from build123d import *

# Parameters (mm, degrees)
F6_R      = 38.8798944489
F7_DEPTH  = 25.146
F9_DEPTH  = 26.67
F10_W     = 18.4118933976
F10_H     = 2.2933566943
F11_DEPTH = 23.368


# Not quite as in the source:
# - a fillet or chamfer that OpenCascade refuses, or shapes differently, is made with other operations: its cross-section is extruded or revolved along the edge and cut away or added


with BuildPart() as f2:
    # F0 (on Front) → F2 (revolve)
    with BuildSketch(Plane.XZ):
        with BuildLine():
            ThreePointArc((-70.200012, 0), (-35.7013462561, 9.759799439), (0, 13.050012))
            Line((0, 13.050012), (0, 19.05))
            ThreePointArc((0, 19.05), (-39.272581084, 14.215324336), (-76.2, 0))
            Line((-76.2, 0), (-70.200012, 0))
        make_face()
    revolve(axis=Axis((0, 0, 24.1573229432), (0, 0, 1)))

    # F3: fillet of radius 2 on 1 edges, made by hand

    # F3_s1 → F3_t2 (revolve, cut)
    with BuildSketch(Plane.XZ):
        with BuildLine():
            ThreePointArc((-69.7074569816, 3.2775780346), (-70.8242638288, 1.7696123233), (-70.200012, 0))
            Line((-70.200012, 0), (-76.2, 0))
            ThreePointArc((-76.2, 0), (-72.9721325586, 1.6752455717), (-69.7074569816, 3.2775780346))
        make_face()
    revolve(axis=Axis((0, 0, 0), (0, 0, 1)), mode=Mode.SUBTRACT)

    # F6 (on offset) → F7 (cut)
    with BuildSketch(Plane.XY.offset(13.0556)):
        Circle(F6_R)
        with BuildLine():
            ThreePointArc((25.4, 0.3187083348), (25.2716745644, -2.231284746), (24.8879949046, -4.7555117659))
            ThreePointArc((24.8879949046, -4.7555117659), (24.4197271347, -6.6696338625), (23.8044800528, -8.5416939933))
            ThreePointArc((23.8044800528, -8.5416939933), (-24.9979378484, 4.8201640248), (25.4, 0.3187083348))
        make_face(mode=Mode.SUBTRACT)
        with BuildLine():
            Line((0, 0.3187083348), (0, 19.3497721271))
            ThreePointArc((0, 19.3497721271), (-19.0310637922, 0.3187083348), (0, -18.7123554574))
            Line((0, -18.7123554574), (0, 0.3187083348))
        make_face()
        with BuildLine():
            Line((0, 19.3497721271), (0, 19.3687083348))
            ThreePointArc((0, 19.3687083348), (13.2989496278, 13.9533806489), (19.0390180892, 0.7913348654))
            ThreePointArc((19.0390180892, 0.7913348654), (19.9506333706, 0.3253641448), (20.8212014385, -0.2134144487))
            ThreePointArc((20.8212014385, -0.2134144487), (20.8263002903, 0.0526252288), (20.828, 0.3187083348))
            ThreePointArc((20.828, 0.3187083348), (-20.7308721477, 2.3278185842), (20.4403944696, -3.6807738728))
            ThreePointArc((20.4403944696, -3.6807738728), (19.6537458396, -3.1118600746), (18.8168844801, -2.6197807703))
            ThreePointArc((18.8168844801, -2.6197807703), (12.3848096584, -14.1516820769), (0, -18.7312916652))
            Line((0, -18.7312916652), (0, -18.7123554574))
            ThreePointArc((0, -18.7123554574), (-19.0310637922, 0.3187083348), (0, 19.3497721271))
        make_face()
        with BuildLine():
            ThreePointArc((0.0092738827, 19.3497698675), (0.0046369415, 19.3497715622), (0, 19.3497721271))
            Line((0, 19.3497721271), (0, 0.3187083348))
            Line((0, 0.3187083348), (0, -18.7123554574))
            ThreePointArc((0, -18.7123554574), (0.0046369415, -18.7123548925), (0.0092738827, -18.7123531978))
            ThreePointArc((0.0092738827, -18.7123531978), (4.4162974191, 0.3187083348), (0.0092738827, 19.3497698675))
        make_face()
        with BuildLine():
            ThreePointArc((13.1388957402, 1.9248430338), (13.7609973094, 1.9418144736), (14.3831748206, 1.9279027252))
            ThreePointArc((14.3831748206, 1.9279027252), (12.1419924656, 8.1965372147), (7.3325286529, 12.7995508523))
            ThreePointArc((7.3325286529, 12.7995508523), (8.9882975444, 0.3187083348), (7.3325286529, -12.1621341826))
            ThreePointArc((7.3325286529, -12.1621341826), (12.0996579985, -7.6240165515), (14.3651267069, -1.4443980064))
            ThreePointArc((14.3651267069, -1.4443980064), (13.9524158986, -1.4394824186), (13.5398409591, -1.4511569053))
            ThreePointArc((13.5398409591, -1.4511569053), (9.5797965511, -0.2096564514), (13.1388957402, 1.9248430338))
        make_face()
    extrude(amount=-F7_DEPTH, mode=Mode.SUBTRACT)

    # F8 (on offset) → F9 (cut)
    with BuildSketch(Plane.XY.offset(18.034)):
        Polygon((-11.6335004568, 11.633916758), (-11.6335004568, 10.6838271022), (0, 10.6838271022), (11.6335004568, 10.6838271022), (11.6335004568, 11.633916758), align=None)
        Polygon((0, 10.6838271022), (-11.6335004568, 10.6838271022), (-11.6335004568, 7.7160974033), (-10.5779496953, 7.7160974033), (-8.4452219732, 7.7160974033), (-7.4719206453, 7.7160974033), (-6.7395351815, 7.7160974033), (0, 7.7160974033), align=None)
        Polygon((11.6335004568, 10.6838271022), (0, 10.6838271022), (0, 7.7160974033), (6.7395351815, 7.7160974033), (7.4719206453, 7.7160974033), (8.4452219732, 7.7160974033), (10.5779496953, 7.7160974033), (11.6335004568, 7.7160974033), align=None)
        Polygon((-10.5779496953, 7.7160974033), (-11.6335004568, 7.7160974033), (-11.6335004568, 7.0042582229), (-10.6457086273, 7.0042582229), align=None)
        Polygon((-8.4452219732, 7.7160974033), (-10.5779496953, 7.7160974033), (-10.6457086273, 7.0042582229), (-8.5129809052, 7.0042582229), align=None)
        Polygon((11.6335004568, 7.0042582229), (11.6335004568, 7.7160974033), (10.5779496953, 7.7160974033), (10.6457086273, 7.0042582229), align=None)
        Polygon((-8.5129809052, 7.0042582229), (-10.6457086273, 7.0042582229), (-11.6335004568, -3.3729556017), (-12.100125514, -8.275069438), (-9.9865486123, -8.4762577367), align=None)
        Polygon((-8.2961780285, -8.637161644), (-6.8072941135, 7.0042582229), (-7.5396795774, 7.0042582229), (-9.0219870399, -8.5680729442), align=None)
        with BuildLine():
            Line((6.8072941135, 7.0042582229), (-6.8072941135, 7.0042582229))
            Line((-6.8072941135, 7.0042582229), (-8.2961780285, -8.637161644))
            add(Edge.make_bspline(
                [(-8.2961780285, -8.637161644), (-5.5307853524, -1.8041071938), (0, 11.8620017068), (5.5307853524, -1.8041071938), (8.2961780285, -8.637161644)],
                knots=[0, 0, 0, 0, 0.5, 1, 1, 1, 1], degree=3))
            Line((8.2961780285, -8.637161644), (6.8072941135, 7.0042582229))
        make_face()
        Polygon((7.5396795774, 7.0042582229), (6.8072941135, 7.0042582229), (8.2961780285, -8.637161644), (9.0219870399, -8.5680729442), align=None)
        Polygon((10.6457086273, 7.0042582229), (10.5779496953, 7.7160974033), (8.4452219732, 7.7160974033), (8.5129809052, 7.0042582229), align=None)
        Polygon((-7.5396795774, 7.0042582229), (-8.5129809052, 7.0042582229), (-9.9865486123, -8.4762577367), (-9.0219870399, -8.5680729442), align=None)
        Polygon((8.5129809052, 7.0042582229), (7.5396795774, 7.0042582229), (9.0219870399, -8.5680729442), (9.9865486123, -8.4762577367), align=None)
        Polygon((11.6335004568, -3.3729556017), (10.6457086273, 7.0042582229), (8.5129809052, 7.0042582229), (9.9865486123, -8.4762577367), (12.100125514, -8.275069438), align=None)
    extrude(amount=F9_DEPTH, mode=Mode.SUBTRACT)

    # F10 (on offset) → F11 (cut)
    with BuildSketch(Plane.XY.offset(18.034)):
        with Locations((-0.0296542421, 7.2142141871)):
            Rectangle(F10_W, F10_H)
    extrude(amount=F11_DEPTH, mode=Mode.SUBTRACT)


solid = f2.part
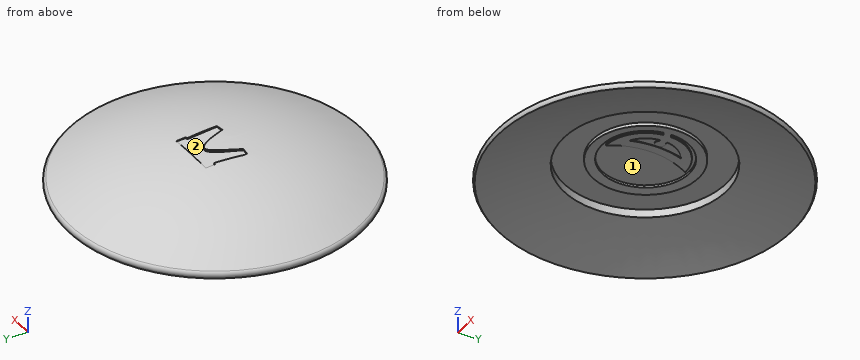
Input: part model. Units: mm. Frame: model coordinates. Face numbers are marked on the shaded views. Give positions to 0.01 mm unless a question says otherwise; leave off trailing zeros. Loops run counter-clockwise (first coordinate to the right, second up) from the corner with the lowest first, then second, coordinate; pieces in that order, holes last. Notation, with made-up numbers: (81, 62) - (140, 62) arc R29 cw to (140, 91) - close; hole circle Ø4 at (39, 8). An arc over 180 degrees is marked (long way). Use CSV: the item, a comma, the result in double quotes. Start each with the question number.
Item 1: Line query: line 1 (Z direction, x = 40, y = 7); line 2 (Z direction, x = 40, y = 57). Output: solid intervals per line, ascending.
Item 2: Section A-A on z = 5. Return loops of the section in (x, y).
Item 3: Mould query, pull axis Y, two halves, no side actions, for the marked faces 1 and 2. Classes: pulls with the +Y half, pulls with the -Y half, needs draft (parallel to the pull), parting line crosses it, or undercut.
Item 4: Contact query for flat-ended pins moving along their axis: P1, Ø1.5, axis at x = -44, z = 2.5, coming from the -Y side; P2, Ø12.5, axis at x = 3, y = 4.5, coming from the -Z side; P3, Ø2, axis at x = 11.5, y = -1.5, coming from the -Z side. Output: stop coordinate, or through.
Ans:
1,line 1,"z = 8.78 to 13.88"
1,line 2,"z = 0.22 to 3.31"
2,outline,"circle Ø131.95 at (0, 0); hole circle Ø111 at (0, 0)"
3,face 1,"undercut"
3,face 2,"undercut"
4,P1,"stops at y = -55.9"
4,P2,"stops at z = 12.7"
4,P3,"stops at z = 12.64"
